from build123d import *

# Parameters (mm, degrees)
F0_R     = 25
F1_DEPTH = 600
F2_T     = -3
F3_R     = 75
F4_DEPTH = 3
F5_W     = 400
F5_H     = 400
F6_DEPTH = 16


# Not quite as in the source:
# - a feature names something its author has since deleted; it is built from what else it names


with BuildPart() as f1:
    # F0 (on Top) → F1 (new body)
    with BuildSketch(Plane.XY):
        Circle(F0_R)
    extrude(amount=F1_DEPTH)

    # F2
    f2_openings = [f1.faces().sort_by_distance(p)[0] for p in [
        (0, 0, 600),
        (0, 0, 0),
    ]]
    offset(amount=F2_T, openings=f2_openings)

    # F3 (on Top) → F4 (join)
    with BuildSketch(Plane.XY):
        Circle(F3_R)
    extrude(amount=F4_DEPTH)

    # F5 (on Top) → F6 (join)
    with BuildSketch(Plane.XY):
        with Locations((125, 125)):
            Rectangle(F5_W, F5_H)
    extrude(amount=-F6_DEPTH)


solid = f1.part
The model under review builds one solid part; all positions refer to its coordinate system, in mm. A direction names the side the tool comes from. Round coordinates to 2 decimals unless told otherwise and drop trailing zeros. Write each loop counter-clockwise with the first axis right and the second up, starting at its lowest first coordinate (ties: lowest second). Pieces come first, ordered by that corner, then holes. Notation, with made-up numbers: M -17,80.5 L 6,80.5 A13 ccw 6,85.5 Z; hole C 73.25,-14.75 d9. An arc over 180 degrees is marked long. Answer as CSV lines item,"result". Start each with the question number.
Q1. The part is to be moulded in two halves that separate along Y. For faces 1 (the face through (122, 325, -8)), 2 (the face through (-4.769, -21.477, 297.321)), 3 (the face through (1.7, -22.1, 600)), 4 (the face through (122, -75, -8)), say which applies: +Y half, -Y half, draft (parallel to the pull), parting line (faces both ways), or undercut.
Q2. Wall thickness on line 1 along X through (y, z) = (0, 387); line 2 along Y through (x, z) = (-2, 54): over which ranges is each line inside the solid? List them lowest first.
Q3. Consider section A-A, the plane z = 383.5. Give the boundary of the cut face in (x, y).
Q4. Consider section D-D, the plane y = -41. Give the boundary of the cut face in (x, z), then the cut area to 3 significant figures.
Q5. Consider section B-B, the plane y = 53. Give the boundary of the cut face in (x, z), then the cut area to 3 significant figures.
Q6. Tool access review of faces 5 (the face through (325, 122, -8)), 6 (the face through (-9.764, 74.362, 1.479)), 7 (the face through (-60, -57, 0)): name each direction out of +Z, -Z, +X, -X, +Y, -Y from which nothing blocks a thin tool from reaching the whole face with its end or side.
Q7. Consider section C-C, the plane x = 202. Give the boundary of the cut face in (y, z), then the cut area to 3 significant figures.
Q8. Clearance check with flat-ended pins moving along their axes: P1, Ø1, axis at x = 232.5, y = 186.5, coming from the +Z side; P2, Ø5, axis at y = -0.5, z = 168.5, coming from the -X side; P3, Ø3, axis at y = -6, z = 187.5, coming from the -X side. State where each tip first meets the part, or that it passes through.
Result set:
1,face 1,"+Y half"
1,face 2,"undercut"
1,face 3,"draft"
1,face 4,"-Y half"
2,line 1,"x = -25 to -22, 22 to 25"
2,line 2,"y = -24.92 to -21.91, 21.91 to 24.92"
3,outline,"C 0,0 d50; hole C 0,0 d44"
4,outline,"M -75,-16 L 325,-16 L 325,0 L 62.8,0 L 62.8,3 L -62.8,3 L -62.8,0 L -75,0 Z"
4,area,"6,780 mm²"
5,outline,"M -75,-16 L 325,-16 L 325,0 L 53.07,0 L 53.07,3 L -53.07,3 L -53.07,0 L -75,0 Z"
5,area,"6,720 mm²"
6,face 5,"+Z, -Z, +X, +Y, -Y"
6,face 6,"+Z"
6,face 7,"+Z, -X, -Y"
7,outline,"M -75,-16 L 325,-16 L 325,0 L -75,0 Z"
7,area,"6,400 mm²"
8,P1,"stops at z = 0"
8,P2,"stops at x = -25"
8,P3,"stops at x = -24.59"
